from build123d import *

# Parameters (mm, degrees)
SKETCH1_R           = 54.9275
SKETCH1_R_2         = 12.7
BOSS_EXTRUDE1_DEPTH = 6.35
SKETCH2_R           = 26.5
CUT_EXTRUDE1_DEPTH  = 1.190625
SKETCH3_R           = 19
CUT_EXTRUDE2_DEPTH  = 2.38125
SKETCH4_R           = 1.4732
CUT_EXTRUDE3_DEPTH  = 7.35


with BuildPart() as part:
    # Sketch1 → Boss-Extrude1 (new body)
    with BuildSketch(Plane(origin=(0, 0, 0), x_dir=(1, 0, 0), z_dir=(0, 1, 0))):
        with Locations(Location((0, 0, 0), (0, 0, 270))):  # turned: the seam where the file's is
            Circle(SKETCH1_R)
        with Locations(Location((0, 0, 0), (0, 0, 270))):  # turned: the seam where the file's is
            Circle(SKETCH1_R_2, mode=Mode.SUBTRACT)
    extrude(amount=BOSS_EXTRUDE1_DEPTH)

    # Sketch2 → Cut-Extrude1 (cut)
    with BuildSketch(Plane(origin=(0, 6.35, 0), x_dir=(1, 0, 0), z_dir=(0, 1, 0))):
        with Locations(Location((0, 0, 0), (0, 0, 270))):  # turned: the seam where the file's is
            Circle(SKETCH2_R)
    extrude(amount=-CUT_EXTRUDE1_DEPTH, mode=Mode.SUBTRACT)

    # Sketch3 → Cut-Extrude2 (cut)
    with BuildSketch(Plane(origin=(0, 6.35, 0), x_dir=(1, 0, 0), z_dir=(0, 1, 0))):
        with Locations(Location((0, 0, 0), (0, 0, 270))):  # turned: the seam where the file's is
            Circle(SKETCH3_R)
    extrude(amount=-CUT_EXTRUDE2_DEPTH, mode=Mode.SUBTRACT)

    # Sketch4 → Cut-Extrude3 (cut, through all)
    with BuildSketch(Plane(origin=(0, 6.35, 0), x_dir=(-1, 0, 0), z_dir=(0, 1, 0))):
        with Locations(Location((-38.1, 0, 0), (0, 0, 90))):  # turned: the seam where the file's is
            Circle(SKETCH4_R)
        with Locations(Location((0, -38.1, 0), (0, 0, 90))):  # turned: the seam where the file's is
            Circle(SKETCH4_R)
        with Locations(Location((38.1, 0, 0), (0, 0, 90))):  # turned: the seam where the file's is
            Circle(SKETCH4_R)
        with Locations(Location((0, 38.1, 0), (0, 0, 90))):  # turned: the seam where the file's is
            Circle(SKETCH4_R)
    extrude(amount=-CUT_EXTRUDE3_DEPTH, mode=Mode.SUBTRACT)


solid = part.part
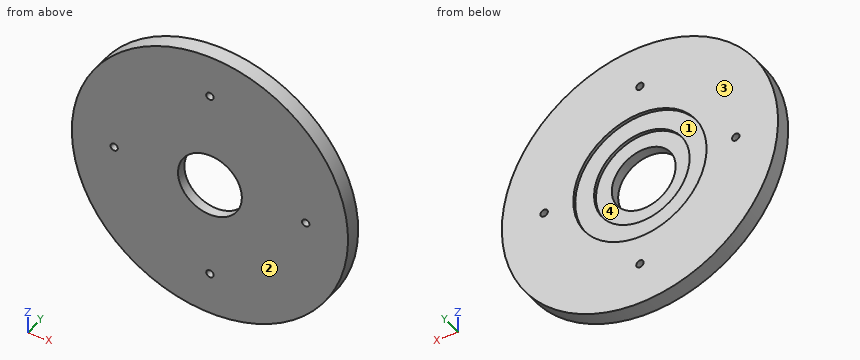
Design review of the part built by this model. Coordinates are the model's own, in mm. Face numbers are marked on the shaded views. A direction names the side the tool comes from. Coordinates: 2 decimals unless noted, no trailing zeros. Loops run counter-clockwise (first coordinate to the right, second up) from the corner with the lowest first, then second, coordinate; pieces in that order, holes last. Notation, with made-up numbers: (36.25, 19) -> (46.25, 19) arc R22 ccw to (46.25, 46) -> close; hole circle Ø7 at (13.5, 45.5). An arc over 180 degrees is marked (long way). Use a Markdown table: item, result. Add a question column.
Item 1: We need section D-D, the plane x = -38.1. Write out the cut boundary in (y, z).
Item 2: Wall thickness on L1, parallel to X at y = 4.2, z = 0; L2, parallel to X at y = 2.9, z = 0; L3, parallel to X at y = 3.5, z = -38.1: over which ranges is each line inside the solid? List them lowest first. Write a range as from..to.
Item 3: The part is to be moulded in two halves that separate along Z. For the marked faces 3 and 4, say which applies: +Z half, -Z half, draft (parallel to the pull), parting line (faces both ways), or undercut.
Item 4: Clearance check with flat-ended pins moving along their axes: P1, Ø3, axis at x = -2.5, y = 3.5, coming from the -Z side; P2, Ø16, axis at x = 6, z = 10, coming from the +Y side. State where each tip first meets the part, or that it passes through.
Item 5: We need section B-B, the plane x = 0. Write out the cut boundary in (y, z).
Item 6: We need section C-C, the plane y = 2.5. Write out the cut boundary in (x, z) (1 decimal).
Item 7: Machinability: for the marked faces 1 and 2, which of the approach directions +Z, -Z, +X, -X, +Y, -Y give a long, thin tool a straight path to every point of the face, cutting with its end or side? Answer none if there is none.
Item 8: We need section A-A, the plane z = 0. Write out the cut boundary in (x, y), and give its area (3 significant figures).
Numbers:
| question | item | result |
|---|---|---|
| 1 | outline | (0, -39.57) -> (6.35, -39.57) -> (6.35, -1.47) -> (0, -1.47) -> close; (0, 1.47) -> (6.35, 1.47) -> (6.35, 39.57) -> (0, 39.57) -> close |
| 2 | L1 | x = -54.93..-39.57, -36.63..-19, 19..36.63, 39.57..54.93 |
| 2 | L2 | x = -54.93..-39.57, -36.63..-12.7, 12.7..36.63, 39.57..54.93 |
| 2 | L3 | x = -39.57..-1.47, 1.47..39.57 |
| 3 | face 3 | draft |
| 3 | face 4 | undercut |
| 4 | P1 | stops at z = -54.92 |
| 4 | P2 | stops at y = 5.16 |
| 5 | outline | (0, -54.93) -> (6.35, -54.93) -> (6.35, -39.57) -> (0, -39.57) -> close; (0, -36.63) -> (6.35, -36.63) -> (6.35, -26.5) -> (5.16, -26.5) -> (5.16, -19) -> (3.97, -19) -> (3.97, -12.7) -> (0, -12.7) -> close; (0, 12.7) -> (3.97, 12.7) -> (3.97, 19) -> (5.16, 19) -> (5.16, 26.5) -> (6.35, 26.5) -> (6.35, 36.63) -> (0, 36.63) -> close; (0, 39.57) -> (6.35, 39.57) -> (6.35, 54.93) -> (0, 54.93) -> close |
| 6 | outline | circle Ø109.9 at (0, 0); hole circle Ø2.9 at (-38.1, 0); hole circle Ø25.4 at (0, 0); hole circle Ø2.9 at (0, -38.1); hole circle Ø2.9 at (0, 38.1); hole circle Ø2.9 at (38.1, 0) |
| 7 | face 1 | +Y |
| 7 | face 2 | +Z, -Z, +X, -X, -Y |
| 8 | outline | (-54.93, 0) -> (-39.57, 0) -> (-39.57, 6.35) -> (-54.93, 6.35) -> close; (-36.63, 0) -> (-12.7, 0) -> (-12.7, 3.97) -> (-19, 3.97) -> (-19, 5.16) -> (-26.5, 5.16) -> (-26.5, 6.35) -> (-36.63, 6.35) -> close; (12.7, 0) -> (36.63, 0) -> (36.63, 6.35) -> (26.5, 6.35) -> (26.5, 5.16) -> (19, 5.16) -> (19, 3.97) -> (12.7, 3.97) -> close; (39.57, 0) -> (54.93, 0) -> (54.93, 6.35) -> (39.57, 6.35) -> close |
| 8 | area | 451 mm^2 |
